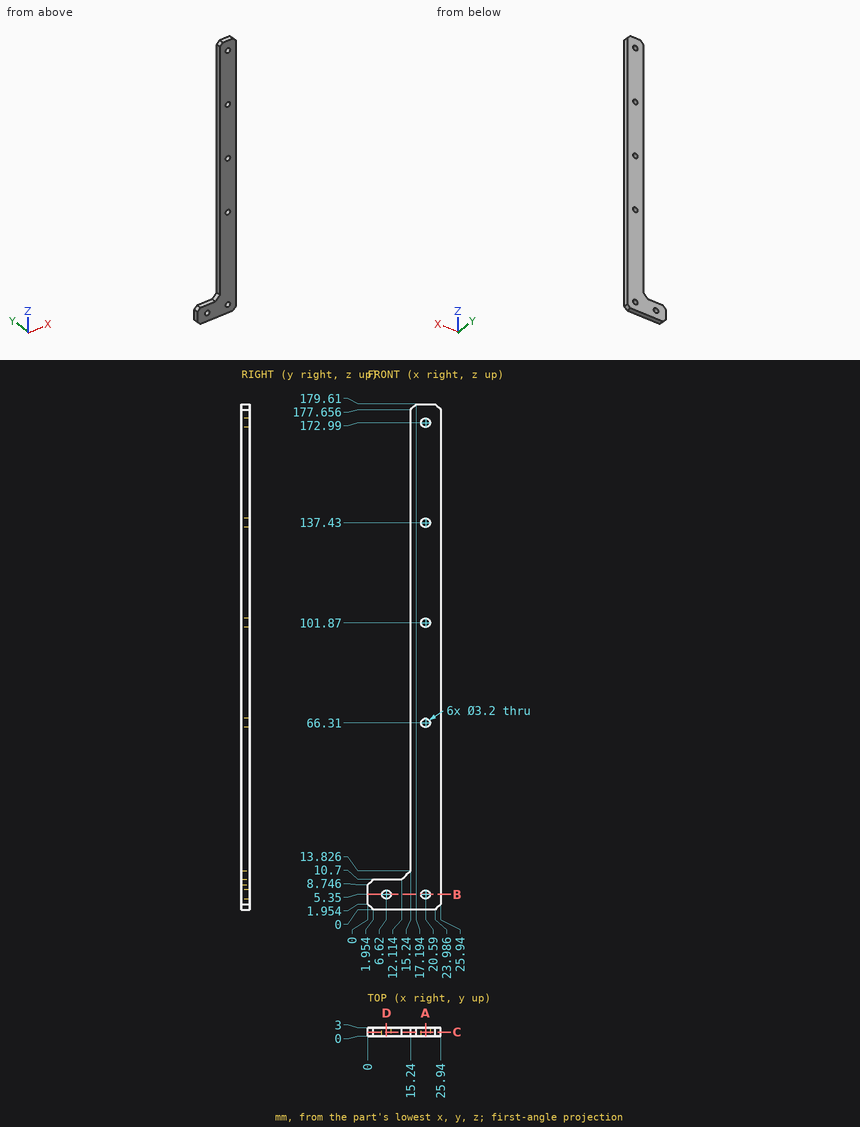
Print and shaded views of the part. All mm, measured from the part's lowest x, y and z. Round coordinates to 2 decimals unless told otherwise and drop trailing zeros. Write each loop counter-clockwise with the first axis right and the second up, starting at its lowest first coordinate (ties: lowest second). Pieces come first, ordered by that corner, then holes. Notation, with made-up numbers: (30.5, 10) -> (45.5, 10) arc R30 ccw to (45.5, 32) -> close; hole circle Ø11 at (40, -12). An arc over 180 degrees is marked (long way). Write item = value, one per line.
(1) Band-saw the part on A-A (x = 20.59). Give the cut face in (y, z).
Answer:
outline = (0, 0) -> (3, 0) -> (3, 3.75) -> (0, 3.75) -> close; (0, 6.95) -> (3, 6.95) -> (3, 64.71) -> (0, 64.71) -> close; (0, 67.91) -> (3, 67.91) -> (3, 100.27) -> (0, 100.27) -> close; (0, 103.47) -> (3, 103.47) -> (3, 135.83) -> (0, 135.83) -> close; (0, 139.03) -> (3, 139.03) -> (3, 171.39) -> (0, 171.39) -> close; (0, 174.59) -> (3, 174.59) -> (3, 179.61) -> (0, 179.61) -> close
(2) Band-saw the part on C-C (y = 1.4). Give the cut face in (x, z), then the cut area to 3 significant figures.
Answer:
outline = (0, 1.95) -> (1.95, 0) -> (23.99, 0) -> (25.94, 1.95) -> (25.94, 177.66) -> (23.99, 179.61) -> (17.19, 179.61) -> (15.24, 177.66) -> (15.24, 13.83) -> (12.11, 10.7) -> (1.95, 10.7) -> (0, 8.75) -> close; hole circle Ø3.2 at (6.62, 5.35); hole circle Ø3.2 at (20.59, 5.35); hole circle Ø3.2 at (20.59, 66.31); hole circle Ø3.2 at (20.59, 101.87); hole circle Ø3.2 at (20.59, 137.43); hole circle Ø3.2 at (20.59, 172.99)
area = 2,030 mm2
(3) Probe L1, parallel to Z at x = 6.62, y = 1.1; L2, parallel to X at y = 1.8, z = 137.43; L3, parallel to X at y = 1.5, z = 76.5. List the from-to ranges inside material, lowest first.
Answer:
L1 = 0 to 3.75, 6.95 to 10.7
L2 = 15.24 to 18.99, 22.19 to 25.94
L3 = 15.24 to 25.94
(4) Band-saw the part on D-D (x = 6.62). Give the cut face in (y, z), then the cut area to 3 significant figures.
Answer:
outline = (0, 0) -> (3, 0) -> (3, 3.75) -> (0, 3.75) -> close; (0, 6.95) -> (3, 6.95) -> (3, 10.7) -> (0, 10.7) -> close
area = 22.5 mm2
(5) Flat gauge pins, fed straight in: pin 1 (4 mm diameter, centred on x = 20.59, z = 101.87, fed in from -Y); pin 2 (1.9 mm diameter, centred on x = 20.59, z = 66.31, fed in from -Y). Where does each tip first touch, or does it go through?
Answer:
pin_1 = 0
pin_2 = through
(6) Band-saw the part on B-B (z = 5.35). Give the cut face in (x, y).
Answer:
outline = (0, 0) -> (5.02, 0) -> (5.02, 3) -> (0, 3) -> close; (8.22, 0) -> (18.99, 0) -> (18.99, 3) -> (8.22, 3) -> close; (22.19, 0) -> (25.94, 0) -> (25.94, 3) -> (22.19, 3) -> close
